Verification items for this drawing (mm, ordinates from the low corner). A direction names the side the tool comes from. Give positions to 0.01 mm unless a question says otherwise; leave off trailing zeros. Write each loop counter-clockwise with the first axis right and the second up, starting at its lowest first coordinate (ties: lowest second). Pieces come first, ordered by that corner, then holes. Notation, with made-up numbers: (-34.5, -13.75) -> (21.5, -13.75) arc R22 ccw to (21.5, 25.25) -> close; hole circle Ø1 at (71, 5). An arc over 180 degrees is marked (long way). Use one line per item in the form item = value. Start each with the question number.
(1) Section check A-A, the plane z = 32. Record the cut outline in (x, y), plus the area to 3 significant figures.
(2) Depth check by flat-ended pin: pin 1 Ø1 at (y, z) = (20.5, 32) entering from -X; pin 2 Ø10 at (x, z) = (3, 10) entering from +Y; pin 3 Ø10 at (y, z) = (14, 15.5) entering from -X. Enter the tip coordinate at first touch or a pass-through.
(3) Scan lines: L1, parallel to Y at x = 13, z = 13; L2, parallel to Z at x = 4.5, y = 9.25. Record each from-to range of solid material in increasing order.
(4) Section check B-B, the plane z = 51. Record the cut outline in (x, y).
(5) Set-up check for the marked faces 4 and 5: record each of +Z, -Z, +X, -X, +Y, -Y from which the full face is reachable in a straight line by a thin tool's end or side.
(6) Release check for a two-part mould opening along Y. For the marked faces 1, 2 and 3 record: pulls with the +Y half, pulls with the -Y half, needs draft (parallel to the pull), parting line crosses it, or undercut.
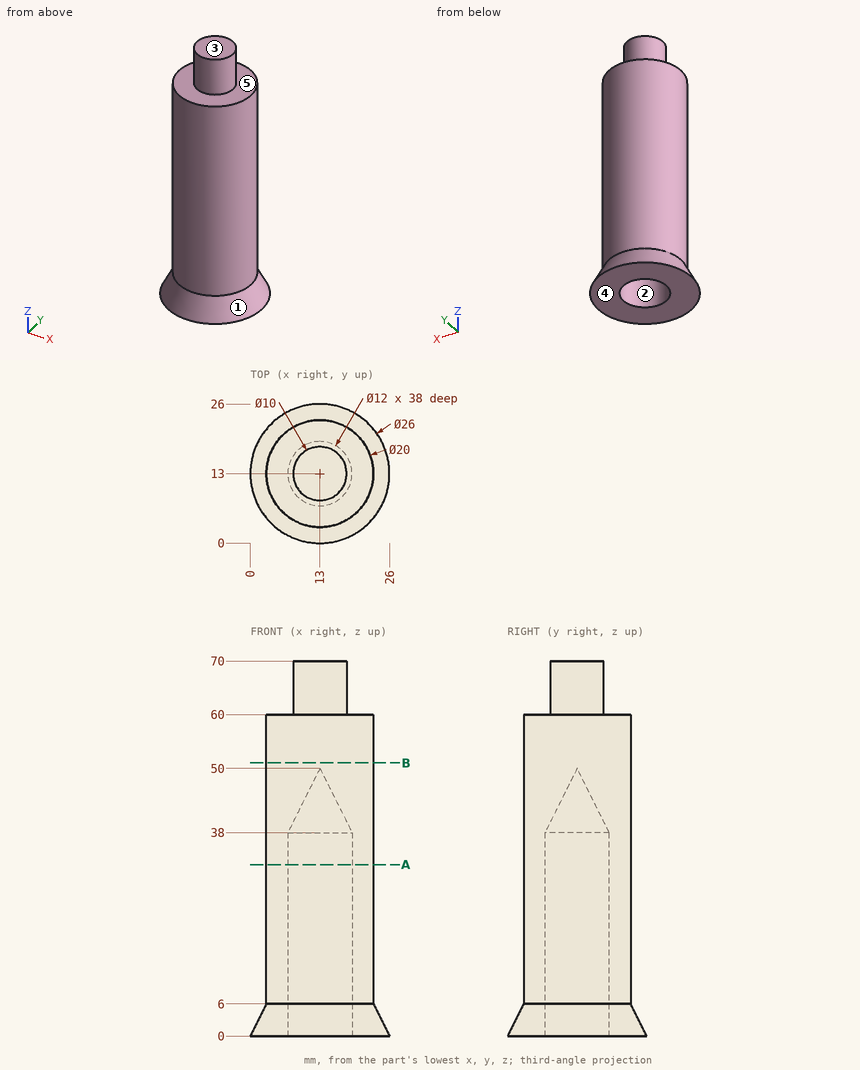
Completed:
q1.outline = circle Ø20 at (13, 13); hole circle Ø12 at (13, 13)
q1.area = 201 mm²
q2.pin_1 = 5.86
q2.pin_2 = 21.66
q2.pin_3 = 3
q3.L1 = 3 to 7, 19 to 23
q3.L2 = 0 to 60
q4.outline = circle Ø20 at (13, 13)
q5.face_4 = -Z, +X, -X, +Y, -Y
q5.face_5 = +Z
q6.face_1 = parting line crosses it
q6.face_2 = undercut
q6.face_3 = needs draft
